from build123d import *

# Parameters (mm, degrees)
BOSS_EXTRUDE1_DEPTH = 300
SKETCH2_W           = 142.5
SKETCH2_H           = 65
SKETCH2_H_2         = 92.5
SKETCH2_H_3         = 22.5
SKETCH2_H_4         = 2.5
CUT_EXTRUDE1_DEPTH  = 69
SKETCH3_W           = 142.5
SKETCH3_H           = 26
SKETCH3_W_2         = 290
SKETCH3_H_2         = 40
CUT_EXTRUDE2_DEPTH  = 195
BOSS_EXTRUDE2_DEPTH = 290
FILLET1_R           = 2
FILLET2_R           = 5


with BuildPart() as part:
    # Sketch1 → Boss-Extrude1 (new body)
    with BuildSketch(Plane(origin=(0, 0, 0), x_dir=(0, 0, -1), z_dir=(1, 0, 0))):
        with BuildLine():
            Line((-96.96969697, -62.878787879), (103.03030303, -62.878787879))
            Line((103.03030303, -62.878787879), (103.03030303, 87.121212121))
            Line((103.03030303, 87.121212121), (3.03030303, 87.121212121))
            ThreePointArc((3.03030303, 87.121212121), (-67.680375088, 57.83189024), (-96.96969697, -12.878787879))
            Line((-96.96969697, -12.878787879), (-96.96969697, -62.878787879))
        make_face()
    extrude(amount=-BOSS_EXTRUDE1_DEPTH)

    # Sketch2 → Cut-Extrude1 (cut)
    with BuildSketch(Plane(origin=(0, 87.121212121, 0), x_dir=(1, 0, 0), z_dir=(0, 1, 0))):
        with Locations((-223.75, 65.53030303)):
            Rectangle(SKETCH2_W, SKETCH2_H)
        with Locations((-76.25, 51.78030303)):
            Rectangle(SKETCH2_W, SKETCH2_H_2)
        with Locations((-76.25, -45.71969697)):
            Rectangle(SKETCH2_W, SKETCH2_H_2)
        with Locations((-223.75, -45.71969697)):
            Rectangle(SKETCH2_W, SKETCH2_H_2)
        with Locations((-223.75, 16.78030303)):
            Rectangle(SKETCH2_W, SKETCH2_H_3)
        with Locations((-223.75, 4.28030303)):
            Rectangle(SKETCH2_W, SKETCH2_H_4)
        with Locations((-223.75, 1.78030303)):
            Rectangle(SKETCH2_W, SKETCH2_H_4)
    extrude(amount=-CUT_EXTRUDE1_DEPTH, mode=Mode.SUBTRACT)

    # Sketch3 → Cut-Extrude2 (cut)
    with BuildSketch(Plane.XY.offset(96.96969697)):
        with Locations((-76.25, 0.121212121)):
            Rectangle(SKETCH3_W, SKETCH3_H)
        with Locations((-223.75, 0.121212121)):
            Rectangle(SKETCH3_W, SKETCH3_H)
        with Locations((-150, -37.878787879)):
            Rectangle(SKETCH3_W_2, SKETCH3_H_2)
    extrude(amount=-CUT_EXTRUDE2_DEPTH, mode=Mode.SUBTRACT)

    # Sketch4 → Boss-Extrude2 (add)
    with BuildSketch(Plane(origin=(-295, 0, 0), x_dir=(0, 0, -1), z_dir=(1, 0, 0))):
        with BuildLine():
            Line((-72.769752814, 18.121212121), (-72.769752814, 44.386834741))
            ThreePointArc((-72.769752814, 44.386834741), (-80.804635484, 31.805695829), (-86.769474252, 18.121212121))
            Line((-86.769474252, 18.121212121), (-72.769752814, 18.121212121))
        make_face()
        with BuildLine():
            ThreePointArc((-86.769474252, 18.121212121), (-80.804635484, 31.805695829), (-72.769752814, 44.386834741))
            Line((-72.769752814, 44.386834741), (-77.983342338, 45.745347629))
            ThreePointArc((-77.983342338, 45.745347629), (-86.036408668, 32.586813044), (-91.96969697, 18.346202113))
            Line((-91.96969697, 18.346202113), (-91.96969697, 18.121212121))
            Line((-91.96969697, 18.121212121), (-86.769474252, 18.121212121))
        make_face()
    extrude(amount=BOSS_EXTRUDE2_DEPTH)

    # Fillet1
    fillet1_edges = [part.edges().sort_by_distance(p)[0] for p in [
        (-300, 12.121212121, -103.03030303),
        (-300, 87.121212121, -53.03030303),
        (-300, 57.83189024, 67.680375088),
        (-300, -37.878787879, 96.96969697),
        (0, 57.83189024, 67.680375088),
        (0, 87.121212121, -53.03030303),
        (0, 12.121212121, -103.03030303),
        (0, -37.878787879, 96.96969697),
    ]]
    fillet(fillet1_edges, radius=FILLET1_R)

    # Fillet2
    fillet2_edges = [part.edges().sort_by_distance(p)[0] for p in [
        (-5, 45.066091185, 75.376547576),
        (-295, 45.066091185, 75.376547576),
    ]]
    fillet(fillet2_edges, radius=FILLET2_R)


solid = part.part
Read the model definition and answer for the solid it produces. Units are mm, in the model's axes. A direction names the side the tool comes from. Round coordinates to 2 decimals unless told otherwise and drop trailing zeros. Loops run counter-clockwise (first coordinate to the right, second up) from the corner with the lowest first, then second, coordinate; pieces in that order, holes last.
Q1. Consider probe 1 along Y at (x, z) = (-208, 40.5); probe 2 along X at (y, z) = (-4, 69); probe 3 along Y at (x, z) = (-225.5, -29.5). Determine where each line is inside the solid, lowest interval first.
Q2. Section B-B on x = -235.5 is taken. Write down the section's boundary in (y, z), and give its area (3 significant figures).
Q3. Section A-A on z = -84 is taken. Write down the section's boundary in (x, y), and give its area (3 significant figures).
Q4. Section D-D on x = -132.5 is taken. Write down the section's boundary in (y, z).
Q5. Determine the mould class of faces 4 (the face through (-77, 34, 72.77)), 5 (the face through (-225, 0, -98.03)), 6 (the face through (-147.928, 45.376, 78.249)) for opening direction Y: released by +Y, released by -Y, zero draft, split by the parting line, or undercut.
Q6. Which of the six approach directions +Z, -Z, +X, -X, +Y, -Y give full straight-line access (tool end or side, diameter ignored) to faces 1 (the face through (-149.3, -58.1, 96.97)), 2 (the face through (-77, 0, -98.03)), 3 (the face through (-225, 53, -28.03))?
Q7. Section C-C on y = -47 is taken. Write down the section's boundary in (x, z), and give its area (3 significant figures).
Q8. Each of these flat-tipped pins is pushed along its axis until it touches: pin 1 (2 mm diameter, centred on x = -43.5, z = -23, fed in from +Y); pin 2 (6 mm diameter, centred on x = -151.5, y = 51.5, fed in from +Z); pin 3 (3 mm diameter, centred on x = -67, y = -26.5, fed in from +Z). Where does it stop, or does it pass through?
Output:
1. probe 1: y = -62.88 to -57.88, -17.88 to -12.88, 13.12 to 18.12
1. probe 2: x = -300 to -295, -152.5 to -147.5, -5 to 0
1. probe 3: y = -62.88 to -57.88, -17.88 to -12.88, 13.12 to 87.12
2. outline: (-62.88, -103.03) - (87.12, -103.03) - (87.12, -98.03) - (18.12, -98.03) - (18.12, -33.03) - (87.12, -33.03) - (87.12, -28.03) - (18.12, -28.03) - (18.12, 72.77) - (44.39, 72.77) - (45.75, 77.98) arc R100 ccw to (13.12, 93.53) - (13.12, -98.03) - (-12.88, -98.03) - (-12.88, 96.97) - (-17.88, 96.97) - (-17.88, -98.03) - (-57.88, -98.03) - (-57.88, 96.97) - (-62.88, 96.97) - close
2. area: 4,360 mm2
3. outline: (-300, -62.88) - (0, -62.88) - (0, 85.12) arc R2 ccw to (-2, 87.12) - (-5, 87.12) - (-5, 18.12) - (-147.5, 18.12) - (-147.5, 87.12) - (-152.5, 87.12) - (-152.5, 18.12) - (-295, 18.12) - (-295, 87.12) - (-298, 87.12) arc R2 ccw to (-300, 85.12) - close; hole (-295, -57.88) - (-5, -57.88) - (-5, -17.88) - (-295, -17.88) - close; hole (-295, -12.88) - (-152.5, -12.88) - (-152.5, 13.12) - (-295, 13.12) - close; hole (-147.5, -12.88) - (-5, -12.88) - (-5, 13.12) - (-147.5, 13.12) - close
3. area: 6,320 mm2
4. outline: (-62.88, -103.03) - (87.12, -103.03) - (87.12, -98.03) - (18.12, -98.03) - (18.12, -5.53) - (87.12, -5.53) - (87.12, -3.03) arc R100 ccw to (87.09, -0.53) - (18.12, -0.53) - (18.12, 72.77) - (44.39, 72.77) - (45.75, 77.98) arc R100 ccw to (13.12, 93.53) - (13.12, -98.03) - (-12.88, -98.03) - (-12.88, 96.97) - (-17.88, 96.97) - (-17.88, -98.03) - (-57.88, -98.03) - (-57.88, 96.97) - (-62.88, 96.97) - close
5. face 4: zero draft
5. face 5: undercut
5. face 6: released by +Y
6. face 1: +Z, +X, -X, +Y, -Y
6. face 2: +Z
6. face 3: +Y
7. outline: (-300, -101.03) arc R2 ccw to (-298, -103.03) - (-2, -103.03) arc R2 ccw to (0, -101.03) - (0, 94.97) arc R2 ccw to (-2, 96.97) - (-5, 96.97) - (-5, -98.03) - (-295, -98.03) - (-295, 96.97) - (-298, 96.97) arc R2 ccw to (-300, 94.97) - close
7. area: 3,450 mm2
8. pin 1: stops at y = 18.12
8. pin 2: stops at z = 75.92
8. pin 3: stops at z = -98.03
